Here's how the part is built. I have some questions about the finished solid (model axes, mm). Face numbers are marked on the shaded views. A direction names the side the tool comes from. Round coordinates to 2 decimals unless told otherwise and drop trailing zeros. Order: outer loops, then holes, each group sorted by start corner. A loop starts at its lowest first (then second) coordinate and runs counter-clockwise, first axis right, second up. Notation, with made-up numbers: (59, -7.75) -> (88, -7.75) arc R6 ccw to (88, 1.25) -> close; hole circle Ø10 at (-23.5, -0.75). An arc over 180 degrees is marked (long way). One line per item, written item: value.
```python
from build123d import *

# Parameters (mm, degrees)
ESQUISSE2_R             = 1.5
ENL_V_MAT_EXTRU_1_DEPTH = 16.43534904


with BuildPart() as part:
    # Esquisse1 → Révolution1 (revolve)
    with BuildSketch(Plane.XY, mode=Mode.PRIVATE) as r_volution1_sk:
        Polygon((2.5, -7), (2.5, 10.5), (6.5, 10.5), (6.5, 7), (8, 7), (8, 4), (5.82, 4), (5.82, -4), (8, -4), (8, -7), align=None)
    revolve(r_volution1_sk.sketch.rotate(Axis((0, 5.91926869, 0), (0, -1, 0)), 90), axis=Axis((0, 5.91926869, 0), (0, -1, 0)))

    # Esquisse2 → Enlèv. mat.-Extru.1 (cut, through all)
    with BuildSketch(Plane.XY):
        with Locations((0, 7.5)):
            Circle(ESQUISSE2_R)
    extrude(amount=-ENL_V_MAT_EXTRU_1_DEPTH, mode=Mode.SUBTRACT)


solid = part.part
```
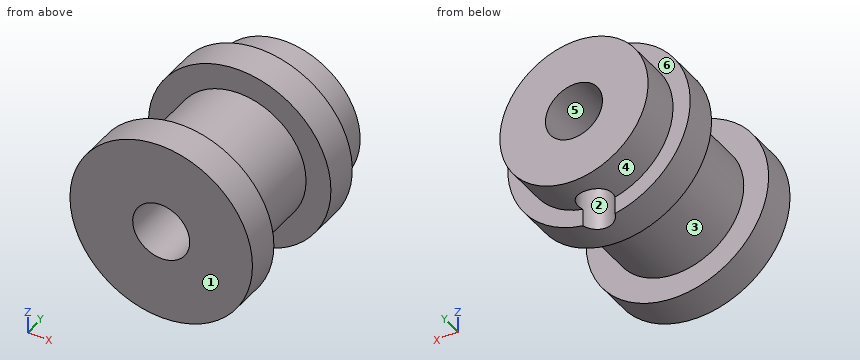
Q1. I want a section at C-C on x = -6.25. Write out the boundary of the cut face in (y, z).
Answers:
outline: (-7, -4.99) -> (-4, -4.99) -> (-4, 4.99) -> (-7, 4.99) -> close; (4, -4.99) -> (7, -4.99) -> (7, -1.79) -> (10.5, -1.79) -> (10.5, 1.79) -> (7, 1.79) -> (7, 4.99) -> (4, 4.99) -> close
Q2. For P1, Ø5, axis at y = 7, z = 5, coming from the +X side; P2, Ø4, axis at y = 3.5, z = 5, coming from the +X side; P3, Ø6, axis at x = -0.5, y = 0, coming from the -Z side; P4, Ø6, axis at x = 1.5, z = -1, coming from the +Y side, each with a flat end and sliding along its axis, tell me the tip position at first contact or that it passes through.
Answers:
P1: x = 7.6
P2: x = 7.39
P3: z = -5.82
P4: y = 10.5
Q3. If we mould it in two halves opening along X, with no side actions, what happens to the marked faces 4, 5 and 6? For each: pulls with the +X half, pulls with the -X half, needs draft (parallel to the pull), parting line crosses it, or undercut.
Answers:
face 4: parting line crosses it
face 5: undercut
face 6: needs draft
Q4. I want a section at B-B on y = -1. Write out the boundary of the cut face in (x, z).
Answers:
outline: circle Ø11.64 at (0, 0); hole circle Ø5 at (0, 0)
Q5. I want a section at A-A on z = 0. Write out the boundary of the cut face in (x, y), then the cut area to 3 significant figures.
Answers:
outline: (-8, -7) -> (-2.5, -7) -> (-2.5, 10.5) -> (-6.5, 10.5) -> (-6.5, 7) -> (-8, 7) -> (-8, 4) -> (-5.82, 4) -> (-5.82, -4) -> (-8, -4) -> close; (2.5, -7) -> (8, -7) -> (8, -4) -> (5.82, -4) -> (5.82, 4) -> (8, 4) -> (8, 7) -> (6.5, 7) -> (6.5, 10.5) -> (2.5, 10.5) -> close
area: 147 mm2
Q6. Which directions (+Z, -Z, +X, -X, +Y, -Y) give clear straight access to the entire face, cutting with the end or side of a thin tool? Please do the marked faces 1, 2 and 3.
Answers:
face 1: +Z, -Z, +X, -X, -Y
face 2: -Z
face 3: none
Q7. I need wall thicknesses on line 1 along X through (y, z) = (6.5, 0); line 2 along Y through (x, z) = (-2.75, -6); line 3 along X through (y, z) = (1.5, 0). Which ranges of each line are inside material? Lowest first, please.
Answers:
line 1: -8 to -2.5, 2.5 to 8
line 2: -7 to -4, 4 to 7
line 3: -5.82 to -2.5, 2.5 to 5.82
Q8. I want a section at D-D on z = -5. Write out the boundary of the cut face in (x, y) (3 decimals).
Answers:
outline: (-6.245, -7) -> (6.245, -7) -> (6.245, -4) -> (2.979, -4) -> (2.979, 4) -> (6.245, 4) -> (6.245, 7) -> (4.153, 7) -> (4.153, 10.5) -> (-4.153, 10.5) -> (-4.153, 7) -> (-6.245, 7) -> (-6.245, 4) -> (-2.979, 4) -> (-2.979, -4) -> (-6.245, -4) -> close; hole circle Ø3 at (0, 7.5)
